The listing builds one solid part. Answer for the finished solid, in the listing's coordinates (mm). Round coordinates to 2 decimals unless told otherwise and drop trailing zeros. Write each loop counter-clockwise with the first axis right and the second up, starting at its lowest first coordinate (ties: lowest second). Pieces come first, ordered by that corner, then holes.
Item 1: Find section B-B on x = 16.92. Give the vertices of the cut face in (y, z), then the cut area to 3 significant figures.
Item 2: Each of these flat-tipped pins is pushed along its axis until it touches: pin 1 (1.5 mm diameter, centred on y = -1, z = -1, fed in from -X); pin 2 (1.1 mm diameter, centred on x = 9, z = -1.5, fed in from +Y). Where does it stop, or does it pass through?
Item 3: Find section C-C on y = 7.75. Give the number of separate pieces and of enclosed holes in the cut face, then the cut area to 3 significant figures.
Item 4: For a pull along Z with two mould halves and no side action, classify faces 1 (the face through (10, 4, 0)), 2 (the face through (9, 3.5, -1)), 3 (the face through (4, 6, -1.75)) as +Z half, -Z half, draft (parallel to the pull), parting line (faces both ways), or undercut.
Item 5: Find section A-A on y = -1. Give the vertices of the cut face in (x, z).
Item 6: Find the intervals of material crossed by probe 1 along Z at (x, y) = (4.5, 6.5); probe 2 along Y at (x, z) = (16.75, -0.15), in increasing order.
```python
from build123d import *

# Parameters (mm, degrees)
SKETCH1_W           = 21
SKETCH1_H           = 2.5
BOSS_EXTRUDE1_DEPTH = 8.5
SKETCH2_W           = 1
SKETCH2_H           = 1
CUT_EXTRUDE1_DEPTH  = 5
CHAMFER1_SIZE       = 0.5
SKETCH4_R           = 0.25
BOSS_EXTRUDE2_DEPTH = 6.5


with BuildPart() as part:
    # Sketch1 → Boss-Extrude1 (new body)
    with BuildSketch(Plane(origin=(0, 0, 0), x_dir=(1, 0, 0), z_dir=(0, 1, 0))):
        with Locations((10.5, 1.25)):
            Rectangle(SKETCH1_W, SKETCH1_H)
    extrude(amount=BOSS_EXTRUDE1_DEPTH)

    # Sketch2 → Cut-Extrude1 (cut)
    with BuildSketch(Plane(origin=(0, 8.5, 0), x_dir=(1, 0, 0), z_dir=(0, 1, 0))):
        with Locations((1.5, 1.25)):
            Rectangle(SKETCH2_W, SKETCH2_H)
        with Locations((4.07, 1.25)):
            Rectangle(SKETCH2_W, SKETCH2_H)
        with Locations((6.64, 1.25)):
            Rectangle(SKETCH2_W, SKETCH2_H)
        with Locations((9.21, 1.25)):
            Rectangle(SKETCH2_W, SKETCH2_H)
        with Locations((11.78, 1.25)):
            Rectangle(SKETCH2_W, SKETCH2_H)
        with Locations((14.35, 1.25)):
            Rectangle(SKETCH2_W, SKETCH2_H)
        with Locations((16.92, 1.25)):
            Rectangle(SKETCH2_W, SKETCH2_H)
        with Locations((19.49, 1.25)):
            Rectangle(SKETCH2_W, SKETCH2_H)
    extrude(amount=-CUT_EXTRUDE1_DEPTH, mode=Mode.SUBTRACT)

    # Chamfer1
    chamfer1_edges = [part.edges().sort_by_distance(p)[0] for p in [
        (1, 8.5, -1.25),
        (1.5, 8.5, -0.75),
        (2, 8.5, -1.25),
        (1.5, 8.5, -1.75),
        (3.57, 8.5, -1.25),
        (4.07, 8.5, -0.75),
        (4.57, 8.5, -1.25),
        (4.07, 8.5, -1.75),
        (6.14, 8.5, -1.25),
        (6.64, 8.5, -0.75),
        (7.14, 8.5, -1.25),
        (6.64, 8.5, -1.75),
        (8.71, 8.5, -1.25),
        (9.21, 8.5, -0.75),
        (9.71, 8.5, -1.25),
        (9.21, 8.5, -1.75),
        (11.28, 8.5, -1.25),
        (11.78, 8.5, -0.75),
        (12.28, 8.5, -1.25),
        (11.78, 8.5, -1.75),
        (13.85, 8.5, -1.25),
        (14.35, 8.5, -0.75),
        (14.85, 8.5, -1.25),
        (14.35, 8.5, -1.75),
        (16.42, 8.5, -1.25),
        (16.92, 8.5, -0.75),
        (17.42, 8.5, -1.25),
        (16.92, 8.5, -1.75),
        (18.99, 8.5, -1.25),
        (19.49, 8.5, -0.75),
        (19.99, 8.5, -1.25),
        (19.49, 8.5, -1.75),
    ]]
    chamfer(chamfer1_edges, length=CHAMFER1_SIZE)

    # Sketch4 → Boss-Extrude2 (add)
    with BuildSketch(Plane(origin=(0, 3.5, 0), x_dir=(1, 0, 0), z_dir=(0, 1, 0))):
        with Locations((1.5, 1.25)):
            Circle(SKETCH4_R)
        with Locations((4.07, 1.25)):
            Circle(SKETCH4_R)
        with Locations((6.64, 1.25)):
            Circle(SKETCH4_R)
        with Locations((9.21, 1.25)):
            Circle(SKETCH4_R)
        with Locations((11.78, 1.25)):
            Circle(SKETCH4_R)
        with Locations((14.35, 1.25)):
            Circle(SKETCH4_R)
        with Locations((16.92, 1.25)):
            Circle(SKETCH4_R)
        with Locations((19.49, 1.25)):
            Circle(SKETCH4_R)
    extrude(amount=-BOSS_EXTRUDE2_DEPTH)


solid = part.part
```
Check values:
1. outline: (-3, -1.5) - (0, -1.5) - (0, -2.5) - (8.5, -2.5) - (8.5, -2.25) - (8, -1.75) - (3.5, -1.75) - (3.5, -0.75) - (8, -0.75) - (8.5, -0.25) - (8.5, 0) - (0, 0) - (0, -1) - (-3, -1) - close
1. area: 17.5 mm2
2. pin 1: stops at x = 1.25
2. pin 2: stops at y = 8.3
3. separate pieces: 1
3. enclosed holes: 8
3. area: 44.5 mm2
4. face 1: +Z half
4. face 2: undercut
4. face 3: undercut
5. outline: circle Ø0.5 at (1.5, -1.25); circle Ø0.5 at (4.07, -1.25); circle Ø0.5 at (6.64, -1.25); circle Ø0.5 at (9.21, -1.25); circle Ø0.5 at (11.78, -1.25); circle Ø0.5 at (14.35, -1.25); circle Ø0.5 at (16.92, -1.25); circle Ø0.5 at (19.49, -1.25)
6. probe 1: z = -2.5 to -1.75, -0.75 to 0
6. probe 2: y = 0 to 8.5
